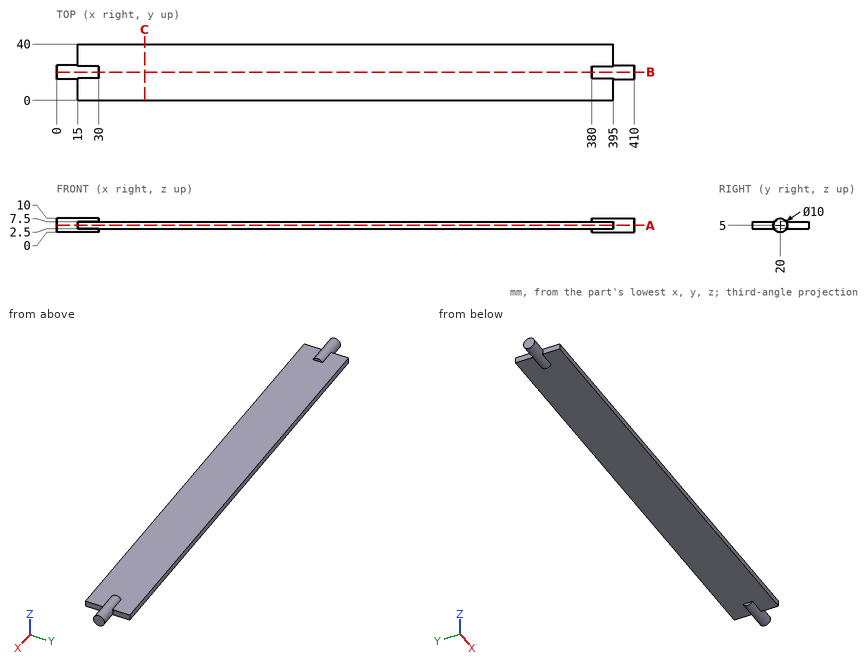
Here's the drawing with two shaded views (mm, measured from the low corner). I have some questions. Round coordinates to 2 decimals unless told otherwise and drop trailing zeros. Loops run counter-clockwise (first coordinate to the right, second up) from the corner with the lowest first, then second, coordinate; pieces in that order, holes last. Notation, with made-up numbers: (87, -3.75) - (98, -3.75) arc R10 cw to (98, 2.25) - close; hole circle Ø2 at (8.25, 84.25). An arc over 180 degrees is marked (long way). Use CSV: the item, a comma, the result in double quotes.
Item 1: I need wall thicknesses on L1, parallel to X at y = 18, z = 8; L2, parallel to Z at x = 107, y = 13.5; L3, parallel to X at y = 30, z = 4.75. Which ranges of each line are inside material? Lowest first, please. Write a range as [from, to].
Here are the results:
L1,"x = [0, 30], [380, 410]"
L2,"z = [2.5, 7.5]"
L3,"x = [15, 395]"
Item 2: If we section it at C-C on x = 62.5: List the corners of the cut face in (y, z) for me, then the cut area to 3 significant figures.
Here are the results:
outline,"(0, 2.5) - (40, 2.5) - (40, 7.5) - (0, 7.5) - close"
area,"200 mm²"
Item 3: If we section it at A-A on z = 5: List the corners of the cut face in (x, y) for me, then the cut area to 3 significant figures.
Here are the results:
outline,"(0, 15) - (15, 15) - (15, 0) - (395, 0) - (395, 15) - (410, 15) - (410, 25) - (395, 25) - (395, 40) - (15, 40) - (15, 25) - (0, 25) - close"
area,"15,500 mm²"
Item 4: Will these pins go through, and if not, where does the flat tip stop? pin 1 (0.8 mm diameter, centred on y = 22, z = 9, fed in from -X); pin 2 (2.5 mm diameter, centred on y = 35.5, z = 5.5, fed in from -X); pin 3 (20 mm diameter, centred on x = 209.5, y = 19, fed in from -Z); pin 4 (5 mm diameter, centred on x = 197, y = 13.5, fed in from +Z).
Here are the results:
pin 1,"stops at x = 0"
pin 2,"stops at x = 15"
pin 3,"stops at z = 2.5"
pin 4,"stops at z = 7.5"
Item 5: If we section it at B-B on y = 20: List the corners of the cut face in (x, z) for me, then the cut area to 3 significant figures.
Here are the results:
outline,"(0, 0) - (30, 0) - (30, 2.5) - (380, 2.5) - (380, 0) - (410, 0) - (410, 10) - (380, 10) - (380, 7.5) - (30, 7.5) - (30, 10) - (0, 10) - close"
area,"2,350 mm²"
